Verification items for the finished model (mm, model axes). Face numbers are marked on the shaded views. Coordinates: 2 decimals unless noted, no trailing zeros. Order: outer loops, then holes, each group sorted by start corner. A loop starts at its lowest first (then second) coordinate and runs counter-clockwise, first axis right, second up.
Q1. Depth check by flat-ended pin: P1, Ø1.5, axis at x = -18.5, z = 227, coming from the -Y side; P2, Ø6, axis at x = 29.5, z = 149, coming from the +Y side; P3, Ø10, axis at x = -93, z = 258, coming from the -Y side. Enter the tip coordinate at first touch or a pass-through.
Q2. Cross-section at A-A, the plane x = 0. Record the boundary of the cut face in (y, z).
Q3. Thickness scan on line 1 (Z direction, x = -116, y = -67); line 2 (Y direction, x = 59, z = 79); line 3 (X direction, y = 33.5, z = 172). Record the ranges inside material, lowest first.
Q4. Cross-section at C-C, the plane z = 164. Record the boundary of the cut face in (x, y).
Q5. Draft check along Z on the marked faces 1, 2, 3 and 4. Enter one of: pulls with the +Z half, pulls with the -Z half, needs draft (parallel to the pull), parting line crosses it, or undercut.
Q6. Cross-section at D-D, the plane x = -119. Record the boundary of the cut face in (y, z), and give its area (3 significant figures).
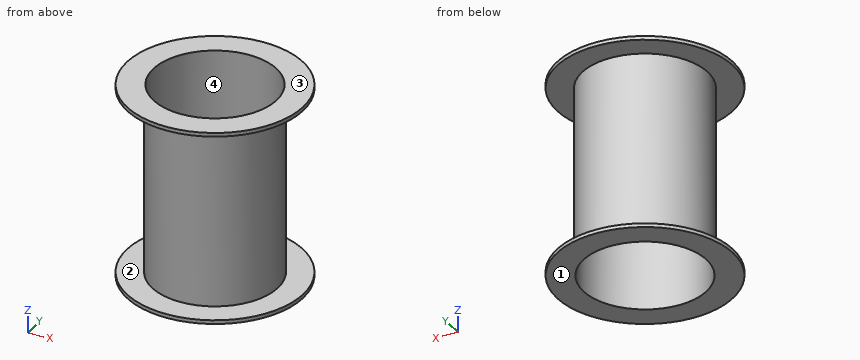
from build123d import *

# Parameters (mm, degrees)
SKETCH1_R           = 100
SKETCH1_R_2         = 98
EXTRUDE_THIN1_DEPTH = 308
SKETCH2_R           = 140
SKETCH2_R_2         = 100
BOSS_EXTRUDE1_DEPTH = 6


with BuildPart() as part:
    # Sketch1 → Extrude-Thin1 (new body)
    with BuildSketch(Plane.XY):
        Circle(SKETCH1_R)
        Circle(SKETCH1_R_2, mode=Mode.SUBTRACT)
    extrude_thin1 = extrude(amount=EXTRUDE_THIN1_DEPTH)

    # Sketch2 → Boss-Extrude1 (add)
    with BuildSketch(Plane.XY.offset(308)):
        Circle(SKETCH2_R)
        Circle(SKETCH2_R_2, mode=Mode.SUBTRACT)
    boss_extrude1 = extrude(amount=-BOSS_EXTRUDE1_DEPTH)

    # Mirror1: Extrude-Thin1, Boss-Extrude1 across plane
    add(extrude_thin1.mirror(Plane(origin=(0, 0, 154), x_dir=(1, 0, 0), z_dir=(0, 0, -1))))
    add(boss_extrude1.mirror(Plane(origin=(0, 0, 154), x_dir=(1, 0, 0), z_dir=(0, 0, -1))))


solid = part.part
Check values:
1. P1: stops at y = -98.41
1. P2: stops at y = 96.42
1. P3: stops at y = -47.5
2. outline: (-140, 0) - (-98, 0) - (-98, 308) - (-140, 308) - (-140, 302) - (-100, 302) - (-100, 6) - (-140, 6) - close; (98, 0) - (140, 0) - (140, 6) - (100, 6) - (100, 302) - (140, 302) - (140, 308) - (98, 308) - close
3. line 1: z = 0 to 6, 302 to 308
3. line 2: y = -80.74 to -78.25, 78.25 to 80.74
3. line 3: x = -94.22 to -92.1, 92.1 to 94.22
4. outline: circle Ø200 at (0, 0); hole circle Ø196 at (0, 0)
5. face 1: pulls with the -Z half
5. face 2: undercut
5. face 3: pulls with the +Z half
5. face 4: needs draft
6. outline: (-73.75, 0) - (73.75, 0) - (73.75, 6) - (-73.75, 6) - close; (-73.75, 302) - (73.75, 302) - (73.75, 308) - (-73.75, 308) - close
6. area: 1,770 mm2
